Could you check a few things on this model? Use its own coordinates, in mm. A direction names the side the tool comes from. Give positions to 0.01 mm unless a question says otherwise; leave off trailing zeros. Write each loop counter-clockwise with the first axis right and the second up, starting at its lowest first coordinate (ties: lowest second). Pieces come first, ordered by that corner, then holes. Notation, with made-up numbers: (-17.75, -35.75) - (0.25, -35.75) arc R26 cw to (0.25, -21.75) - close; hole circle Ø3 at (85, 62). An arc over 180 degrees is marked (long way). Use one line per item in the form item = value.
```python
from build123d import *

# Parameters (mm, degrees)
SKETCH_1_W          = 33
SKETCH_1_H          = 15.6
EXTRUDE_1_DEPTH     = 2
SKETCH_2_W          = 4
SKETCH_2_H          = 3.8
CUT_EXTRUDE_1_DEPTH = 19.360010893
SKETCH_4_W          = 10.8
SKETCH_4_H          = 8
EXTRUDE_2_DEPTH     = 2
EXTRUDE_4_DEPTH     = 8
SKETCH_6_R          = 4
CUT_EXTRUDE_2_DEPTH = 22.20683852
FILLET_1_R          = 2
FILLET_2_R          = 1


with BuildPart() as part:
    # 草图1 → 凸台-拉伸1 (new body)
    with BuildSketch(Plane.XY):
        Rectangle(SKETCH_1_W, SKETCH_1_H)
    extrude(amount=EXTRUDE_1_DEPTH)

    # 草图2 → 切除-拉伸1 (cut, through all)
    with BuildSketch(Plane.XY.offset(2)):
        with Locations((-14.5, 5.9)):
            Rectangle(SKETCH_2_W, SKETCH_2_H)
        with Locations((14.5, 5.9)):
            Rectangle(SKETCH_2_W, SKETCH_2_H)
        with Locations((-14.5, -5.9)):
            Rectangle(SKETCH_2_W, SKETCH_2_H)
        with Locations((14.5, -5.9)):
            Rectangle(SKETCH_2_W, SKETCH_2_H)
    extrude(amount=-CUT_EXTRUDE_1_DEPTH, mode=Mode.SUBTRACT)

    # 草图4 → 凸台-拉伸2 (add)
    with BuildSketch(Plane.ZY.offset(16.5)):
        with Locations((5.4, 0)):
            Rectangle(SKETCH_4_W, SKETCH_4_H)
    extrude_2 = extrude(amount=-EXTRUDE_2_DEPTH)

    # 草图5 → 凸台-拉伸4 (add)
    with BuildSketch(Plane(origin=(0, 4, 0), x_dir=(1, 0, 0), z_dir=(0, 1, 0))):
        with BuildLine():
            Line((-8.45327815, -2.172085136), (-14.5, -8.707152989))
            Line((-14.5, -8.707152989), (-14.5, -10.8))
            ThreePointArc((-14.5, -10.8), (-13.774891977, -10.64781178), (-13.172160334, -10.216931904))
            Line((-13.172160334, -10.216931904), (-6.985279062, -3.530385058))
            Line((-6.985279062, -3.530385058), (-8.45327815, -2.172085136))
        make_face()
    extrude_4 = extrude(amount=-EXTRUDE_4_DEPTH)

    # 草图6 → 切除-拉伸2 (cut, through all)
    with BuildSketch(Plane(origin=(0, 0, 0), x_dir=(-1, 0, 0), z_dir=(0, 0, -1))):
        Circle(SKETCH_6_R)
    extrude(amount=-CUT_EXTRUDE_2_DEPTH, mode=Mode.SUBTRACT)

    # 镜向2: 凸台-拉伸2 across plane
    add(extrude_2.mirror(Plane(origin=(0, 0, 0), x_dir=(0, 0, 1), z_dir=(1, 0, 0))))

    # 镜向3: 凸台-拉伸4 across plane
    add(extrude_4.mirror(Plane(origin=(0, 0, 0), x_dir=(0, 0, 1), z_dir=(1, 0, 0))))

    # 圆角1
    fillet_1_edges = [part.edges().sort_by_distance(p)[0] for p in [
        (16.5, 0, 10.8),
        (-16.5, 0, 10.8),
    ]]
    fillet(fillet_1_edges, radius=FILLET_1_R - 0.0001)  # a hair under: the kernel refuses the full size

    # 圆角2
    fillet_2_edges = [part.edges().sort_by_distance(p)[0] for p in [
        (-16.5, 0, 0),
        (16.5, 0, 0),
    ]]
    fillet(fillet_2_edges, radius=FILLET_2_R)


solid = part.part
```
1. Imagine slicing it at C-C, the plane z = 2.5. List the corners of the cut face in (x, y) for me, and give its area (3 significant figures).
Response values:
outline = (-16.5, -4) - (-14.5, -4) - (-14.5, 4) - (-16.5, 4) - close; (-8.76, -4) - (-8.1, -4) - (-8.1, 4) - (-8.76, 4) - close; (8.1, -4) - (8.76, -4) - (8.76, 4) - (8.1, 4) - close; (14.5, -4) - (16.5, -4) - (16.5, 4) - (14.5, 4) - close
area = 42.5 mm²
2. If I drill on line 1 (Y direction, x = 0, z = 1.6); line 2 (X direction, y = 3.25, z = 6); line 3 (Z direction, x = -4.5, y = 1.75), over which ranges is the centre line in solid material (lowest first)? Write a range as from..to.
Response values:
line_1 = -7.8..-4, 4..7.8
line_2 = -16.5..-14.5, -12..-9.27, 9.27..12, 14.5..16.5
line_3 = 0..2
3. For pin 1 (2 mm diameter, centred on x = 12.5, z = 4.5, fed in from -Y); pin 2 (5 mm diameter, centred on x = -11, z = 5.5, fed in from +Y); pin 3 (3 mm diameter, centred on x = -13, z = 5.5, fed in from -Y); pin 4 (1.6 mm diameter, centred on y = 6, z = 0.5, fed in from +X), each with a flat end and sliding along its axis, tell me the tip position at first contact or that it passes through.
Response values:
pin_1 = through
pin_2 = 4
pin_3 = -4
pin_4 = 12.5
4. Which directions (+Z, -Z, +X, -X, +Y, -Y) give clear straight access to the entire face, cutting with the end or side of a thin tool? Please do faces 5 (the face through (15, 4, 5)), 6 (the face through (10.12, 0.06, 6.92)), 7 (the face through (3, 4, 2)), 8 (the face through (12.5, 6, 1)).
Response values:
face_5 = +Z, +X, +Y
face_6 = +Z, +Y, -Y
face_7 = +Y, -Y
face_8 = +Z, -Z, +X, +Y
5. Imagine slicing it at A-A, the plane x = 0. List the corners of the cut face in (y, z) for me, and give its area (3 significant figures).
Response values:
outline = (-7.8, 0) - (-4, 0) - (-4, 2) - (-7.8, 2) - close; (4, 0) - (7.8, 0) - (7.8, 2) - (4, 2) - close
area = 15.2 mm²
6. If we mould it in two halves opening along Z, with no side actions, what happens to faces 1 (the face through (7.71, 0.06, 2.86)), 2 (the face through (-12.5, -6, 1)), 3 (the face through (13.78, 0.06, 10.65)), 4 (the face through (14.5, 0, 5))? For each: pulls with the +Z half, pulls with the -Z half, needs draft (parallel to the pull), parting line crosses it, or undercut.
Response values:
face_1 = undercut
face_2 = needs draft
face_3 = pulls with the +Z half
face_4 = undercut
